Autodesk Inventor part; units mm, degrees
ref_plane "YZ Plane" through (0, 0, 0) normal (1, 0, 0) x (0, 1, 0)
ref_plane "XZ Plane" through (0, 0, 0) normal (0, 1, 0) x (-1, 0, 0)
ref_plane "XY Plane" through (0, 0, 0) normal (0, 0, 1) x (1, 0, 0)
sketch "Sketch1" plane through (0, 0, 0) normal (0, 0, 1) x (1, 0, 0)
  line L0 (0, 0) -> (22.45, 0)
  line L1 (22.45, 0) -> (22.45, 23.75)
  line L2 (22.45, 23.75) -> (0, 23.75)
  line L3 (0, 23.75) -> (0, 0)
  line L4 (-4.9, 19.45) -> (27.35, 19.45)
  line L5 (27.35, 19.45) -> (27.35, 17)
  line L6 (27.35, 17) -> (-4.9, 17)
  line L7 (-4.9, 17) -> (-4.9, 19.45)
  point P0 (0, 19.45)
  point P1 (0, 17)
  point P2 (22.45, 17)
  point P3 (22.45, 19.45)
  dimension "d0" = 23.75
  dimension "d1" = 22.45
  dimension "d2" = 2.45
  dimension "d3" = 17
  dimension "d4" = 4.9
  dimension "d5" = 4.9
extrude "Extrusion1" add sketch "Sketch1" along normal blind 12
sketch "Sketch2" plane through (22.45, 19.45, 0) normal (0, 1, 0) x (1, 0, 0)
  line L0 (-27.35, 0) -> (-27.35, -12)
  line L1 (-27.35, -6) -> (4.9, -6) construction
  line L2 (4.9, 0) -> (4.9, -12)
  circle A0 centre (-24.975, -6) radius 1.385
  circle A1 centre (2.525, -6) radius 1.385
  circle A2 centre (-24.975, -6) radius 2.375 construction
  circle A3 centre (2.525, -6) radius 2.375 construction
  line L3 (4.9, 0) -> (4.9, -12)
  point P0 (-22.45, 0)
  dimension "d8" = 2.77
  dimension "d9" = 27.5
extrude "Extrusion2" cut sketch "Sketch2" against normal blind 10
sketch "Sketch3" plane through (0, 23.75, 0) normal (0, 1, 0) x (1, 0, 0)
  arc A0 (11.3327, -3.25) -> (11.3327, -8.75) centre (6, -6) ccw
  line L0 (22.45, 0) -> (0, 0)
  line L1 (0, 0) -> (0, -12)
  line L2 (22.45, -12) -> (0, -12)
  arc A1 (11.85, -8.75) -> (11.85, -3.25) centre (11.85, -6) ccw
  line L3 (14.6, -9.3785) -> (14.6, -0.6215) construction
  line L4 (11.85, -6) -> (0, -6) construction
  line L5 (0, 0) -> (0, -12)
  line L6 (11.85, -8.75) -> (11.3327, -8.75)
  line L7 (11.85, -3.25) -> (11.3327, -3.25)
  dimension "d12" = 5.5
  dimension "d13" = 14.6
extrude "Extrusion3" add sketch "Sketch3" along normal blind 4.3 contours L7 A1 L6 A0
sketch "Sketch4" plane through (0, 28.05, 0) normal (0, 1, 0) x (1, 0, 0)
  arc A0 (6, 0) -> (0, -6) centre (6, -6) ccw
  circle A1 centre (6, -6) radius 2.42
  circle A2 centre (6, -6) radius 0.75
  point P0 (0, 0)
  dimension "d16" = 4.84
  dimension "d17" = 1.5
extrude "Extrusion4" add sketch "Sketch4" along normal blind 2.55
properties part number "9g-servo"
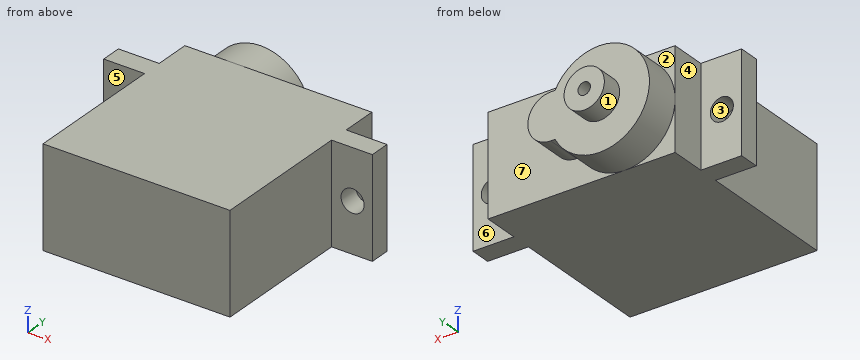
Can you work these out from the model? Positions are in its coordinate system, mm. Face numbers are marked on the shaded views. A direction names the side the tool comes from. Give positions to 0.01 mm unless a question says otherwise; leave off trailing zeros. Loops run counter-clockwise (first coordinate to the right, second up) from the corner with the lowest first, then second, coordinate; pieces in that order, holes last. Notation, with made-up numbers: (69, -4) -> (111, -4) arc R28 cw to (111, 22) -> close; hole circle Ø11 at (47, 20). An arc over 180 degrees is marked (long way). Return JSON: item names as keys, results as strings.
Q1. On a 3-axis mill with a long thin cutter (end or side, diameter ignored), from which of +Z, -Z, +X, -X, +Y, -Y can I reach the whole of each face in a straight line? I mean the marked faces 4, 5, 6 and 7. Say none if no direction works.
Checks:
{"face 4": "+Z, -Z, -X, +Y", "face 5": "+Z, -Z, -X, -Y", "face 6": "+Z, -Z, +X, +Y", "face 7": "+X, +Y"}
Q2. I want a section at B-B, the plane z = 11. List the corners of the cut face in (x, y) for me.
Checks:
{"outline": "(-4.9, 17) -> (0, 17) -> (0, 0) -> (22.45, 0) -> (22.45, 17) -> (27.35, 17) -> (27.35, 19.45) -> (22.45, 19.45) -> (22.45, 23.75) -> (9.32, 23.75) -> (9.32, 28.05) -> (2.68, 28.05) -> (2.68, 23.75) -> (0, 23.75) -> (0, 19.45) -> (-4.9, 19.45) -> close"}
Q3. I want a section at D-D, the plane y = 4. List the corners of the cut face in (x, z) for me.
Checks:
{"outline": "(0, 0) -> (22.45, 0) -> (22.45, 12) -> (0, 12) -> close"}
Q4. For pin 1 Ø5.5 at (x, z) = (26, 4.5) entering from -Y; pin 2 Ø1.3 at (y, z) = (21, 3) entering from -X; pin 3 Ø3.5 at (y, z) = (22.5, 5) entering from +X, each with a flat end and sliding along its axis, tell me the tip position at first contact or that it passes through.
Checks:
{"pin 1": "stops at y = 17", "pin 2": "stops at x = 0", "pin 3": "stops at x = 22.45"}
Q5. We'd pull the mould along X, two halves only. Please class the marked faces 1, 2 and 3: released by +X, released by -X, zero draft, split by the parting line, or undercut.
Checks:
{"face 1": "split by the parting line", "face 2": "zero draft", "face 3": "undercut"}
Q6. I need wall thicknesses on probe 1 along X at (y, z) = (17.85, 6); probe 2 along Z at (x, y) = (6, 29); probe 3 along X at (y, z) = (17.5, 5.5). Which ranges of each line are inside material? Lowest first, please.
Checks:
{"probe 1": "x = -4.9 to -3.91, -1.14 to 23.59, 26.36 to 27.35", "probe 2": "z = 3.58 to 5.25, 6.75 to 8.42", "probe 3": "x = -4.9 to -3.82, -1.23 to 23.68, 26.27 to 27.35"}
Q7. I want a section at C-C, the plane x = 4. List the corners of the cut face in (y, z) for me.
Checks:
{"outline": "(0, 0) -> (23.75, 0) -> (23.75, 0.34) -> (28.05, 0.34) -> (28.05, 4.64) -> (30.6, 4.64) -> (30.6, 7.36) -> (28.05, 7.36) -> (28.05, 11.66) -> (23.75, 11.66) -> (23.75, 12) -> (0, 12) -> close"}
Q8. I want a section at A-A, the plane y = 25. List the corners of the cut face in (x, z) for me, then the cut area to 3 significant figures.
Checks:
{"outline": "(11.33, 3.25) -> (11.85, 3.25) arc R2.75 ccw to (11.85, 8.75) -> (11.33, 8.75) arc R6 ccw (long way) to start", "area": "125 mm2"}
